Check sheet for the modelled part. Datum: model origin and axes. Units: mm. A direction names the side the tool comes from. Round coordinates to 2 decimals unless told otherwise and drop trailing zeros. Loops run counter-clockwise (first coordinate to the right, second up) from the corner with the lowest first, then second, coordinate; pieces in that order, holes last. Notation, with made-up numbers: (22, 30.25) -> (39, 30.25) arc R19 cw to (39, 63.25) -> close; hole circle Ø6 at (-3, 76). An arc over 180 degrees is marked (long way). Return JSON: item names as keys, results as strings.
from build123d import *

# Parameters (mm, degrees)
CROQUIS2_R              = 40.005937341
CROQUIS2_R_2            = 0.995391995
CROQUIS2_R_3            = 1.004055524
CROQUIS2_R_4            = 1.00622676
CROQUIS2_R_5            = 1.004640813
CROQUIS2_R_6            = 1.5
SALIENTE_EXTRUIR1_DEPTH = 2


with BuildPart() as part:
    # Croquis2 → Saliente-Extruir1 (new body)
    with BuildSketch(Plane(origin=(0, 0, 0), x_dir=(1, 0, 0), z_dir=(0, 1, 0))):
        with Locations(Location((0, 0, 0), (0, 0, 270))):
            Circle(CROQUIS2_R)
        with Locations(Location((-31.9766, 9.1, 0), (0, 0, 270))):
            Circle(CROQUIS2_R_2, mode=Mode.SUBTRACT)
        with Locations(Location((-31.9766, -9.1, 0), (0, 0, 270))):
            Circle(CROQUIS2_R_3, mode=Mode.SUBTRACT)
        with Locations(Location((8.2234, 9.1, 0), (0, 0, 270))):
            Circle(CROQUIS2_R_4, mode=Mode.SUBTRACT)
        with Locations(Location((8.2234, -9.1, 0), (0, 0, 270))):
            Circle(CROQUIS2_R_5, mode=Mode.SUBTRACT)
        with Locations(Location((-24.925514037, 24.925514037, 0), (0, 0, 270))):
            Circle(CROQUIS2_R_6, mode=Mode.SUBTRACT)
        with Locations(Location((24.925514037, 24.925514037, 0), (0, 0, 270))):
            Circle(CROQUIS2_R_6, mode=Mode.SUBTRACT)
        with Locations(Location((24.925514037, -24.925514037, 0), (0, 0, 270))):
            Circle(CROQUIS2_R_6, mode=Mode.SUBTRACT)
        with Locations(Location((-24.925514037, -24.925514037, 0), (0, 0, 270))):
            Circle(CROQUIS2_R_6, mode=Mode.SUBTRACT)
        with BuildLine():
            Line((-28.4766, -9.1), (4.7234, -9.1))
            ThreePointArc((4.7234, -9.1), (5.748526266, -6.625126266), (8.2234, -5.6))
            Line((8.2234, -5.6), (8.2234, 5.6))
            ThreePointArc((8.2234, 5.6), (5.748526266, 6.625126266), (4.7234, 9.1))
            Line((4.7234, 9.1), (-28.4766, 9.1))
            ThreePointArc((-28.4766, 9.1), (-29.501726266, 6.625126266), (-31.9766, 5.6))
            Line((-31.9766, 5.6), (-31.9766, -5.6))
            ThreePointArc((-31.9766, -5.6), (-29.501726266, -6.625126266), (-28.4766, -9.1))
        make_face(mode=Mode.SUBTRACT)
        with BuildLine():
            ThreePointArc((-7.653668647, -18.47759065), (0, -20), (7.653668647, -18.47759065))
            ThreePointArc((7.653668647, -18.47759065), (12.553279766, -20.507076026), (10.52379439, -25.406687144))
            ThreePointArc((10.52379439, -25.406687144), (0, -27.5), (-10.52379439, -25.406687144))
            ThreePointArc((-10.52379439, -25.406687144), (-12.553279766, -20.507076026), (-7.653668647, -18.47759065))
        make_face(mode=Mode.SUBTRACT)
        with BuildLine():
            ThreePointArc((-10.52379439, 25.406687144), (-12.553279766, 20.507076026), (-7.653668647, 18.47759065))
            ThreePointArc((-7.653668647, 18.47759065), (0, 20), (7.653668647, 18.47759065))
            ThreePointArc((7.653668647, 18.47759065), (12.553279766, 20.507076026), (10.52379439, 25.406687144))
            ThreePointArc((10.52379439, 25.406687144), (0, 27.5), (-10.52379439, 25.406687144))
        make_face(mode=Mode.SUBTRACT)
    extrude(amount=SALIENTE_EXTRUIR1_DEPTH)


solid = part.part
Q1. Section check A-A (z = 0). Record the boundary of the cut face in (x, y).
Results list:
{"outline": "(-40.01, 0) -> (-31.98, 0) -> (-31.98, 2) -> (-40.01, 2) -> close; (8.22, 0) -> (40.01, 0) -> (40.01, 2) -> (8.22, 2) -> close"}
Q2. Go/stop test with flat-tipped pins: pin 1 (3 mm diameter, centred on x = -31, z = -21, fed in from -Y); pin 2 (1 mm diameter, centred on y = 1, z = -4, fed in from -X); pin 3 (0.6 mm diameter, centred on y = 1, z = -2.5, fed in from +X). Record where each tip stops, or that it passes through.
Results list:
{"pin 1": "y = 0", "pin 2": "x = -39.85", "pin 3": "x = 39.95"}
Q3. Section check C-C (y = 0.4). Count the separate pieces of the cut face and the enclosed holes in it, then the cut area to 3 significant figures.
Results list:
{"separate pieces": "1", "enclosed holes": "11", "area": "3,930 mm^2"}
Q4. Section check B-B (x = 0). Record the boundary of the cut face in (y, z), then the cut area to 3 significant figures.
Results list:
{"outline": "(0, -40.01) -> (2, -40.01) -> (2, -27.5) -> (0, -27.5) -> close; (0, -20) -> (2, -20) -> (2, -9.1) -> (0, -9.1) -> close; (0, 9.1) -> (2, 9.1) -> (2, 20) -> (0, 20) -> close; (0, 27.5) -> (2, 27.5) -> (2, 40.01) -> (0, 40.01) -> close", "area": "93.6 mm^2"}
Q5. Draft check along Z on faces 1 (the flat face through (9, 2, -1)), 2 (the cylindrical face through (-29.475, 0.986, -6.652)). Enter one of: released by +Z, released by -Z, zero draft, split by the parting line, or undercut.
Results list:
{"face 1": "zero draft", "face 2": "undercut"}
Q6. Material ranges on line 1 (Z direction, x = -7, y = 0.1) (3 decimals); line 2 (Z direction, x = -15.5, y = 0.5); line 3 (Z direction, x = -16.5, y = 0.55), recorded low to high.
Results list:
{"line 1": "-39.389 to -26.594, -18.735 to -9.1, 9.1 to 18.735, 26.594 to 39.389", "line 2": "-36.88 to -9.1, 9.1 to 36.88", "line 3": "-36.44 to -9.1, 9.1 to 36.44"}
Q7. Tool access check on faces 3 (the flat face through (-31.977, 1, 0)), 4 (the flat face through (9, 0, -1)). Record the directions out of +Z, -Z, +X, -X, +Y, -Y that give a thin tool (end or side, any length) a straight path to the whole face; none if there is none.
Results list:
{"face 3": "+Y, -Y", "face 4": "+Z, -Z, +X, -X, -Y"}
Q8. Section check D-D (z = 14.5). Record the boundary of the cut face in (x, y), then the cut area to 3 significant figures.
Results list:
{"outline": "(-37.29, 0) -> (37.29, 0) -> (37.29, 2) -> (-37.29, 2) -> close", "area": "149 mm^2"}
